Design review of the part shown in the three views and the two pictorial views. Dimensions are in mm from the part's minimum x, y and z. A direction names the side the tool comes from. Round coordinates to 2 decimals unless told otherwise and drop trailing zeros. Loops run counter-clockwise (first coordinate to the right, second up) from the corner with the lowest first, then second, coordinate; pieces in that order, holes last. Notation, with made-up numbers: M -21.5,68 L 3.5,68 A24 cw 3.5,102 Z; hole C 53,8.25 d4. An arc over 180 degrees is marked long. Return JSON: item names as keys, results as strings. Group by question number.
Q1. Clearance check with flat-ended pins moving along their axes: pin 1 Ø10 at (y, z) = (18.5, 5) entering from -X; pin 2 Ø1 at (x, z) = (5, 35.5) entering from +Y; pin 3 Ø1 at (x, z) = (3.5, 18) entering from -Y; pin 4 Ø3.5 at (y, z) = (19.65, 4.5) entering from -X. State where each tip first meets the part, or that it passes through.
Q2. Consider section D-D (z = 14). State the section outline as (x, y) points, and give its area (3 significant figures).
Q3. For the marked faces 1, 2 and 3, list the 3-axis set-ups (+Z, -Z, +X, -X, +Y, -Y) from which the entire face can be reached by the end or side of a thin tool; tool diameter is ignored.
Q4. Consider section B-B (y = 11.5). State the section outline as (x, z) points.
Q5. Consider section A-A (x = 3). State the section outline as (y, z) points (1 decimal).
Q6. Consider section C-C (y = 18.75). State the section outline as (x, z) points (1 decimal).
Q7. To check wall thickness, follow line 1 along Z through (x, y) = (4.75, 15); line 2 along Y through (x, z) = (5.5, 39) (1 decimal); line 3 along Z through (x, y) = (3.25, 22.25) (1 decimal). State the ranges of each line that lie inside material, in increasing order.
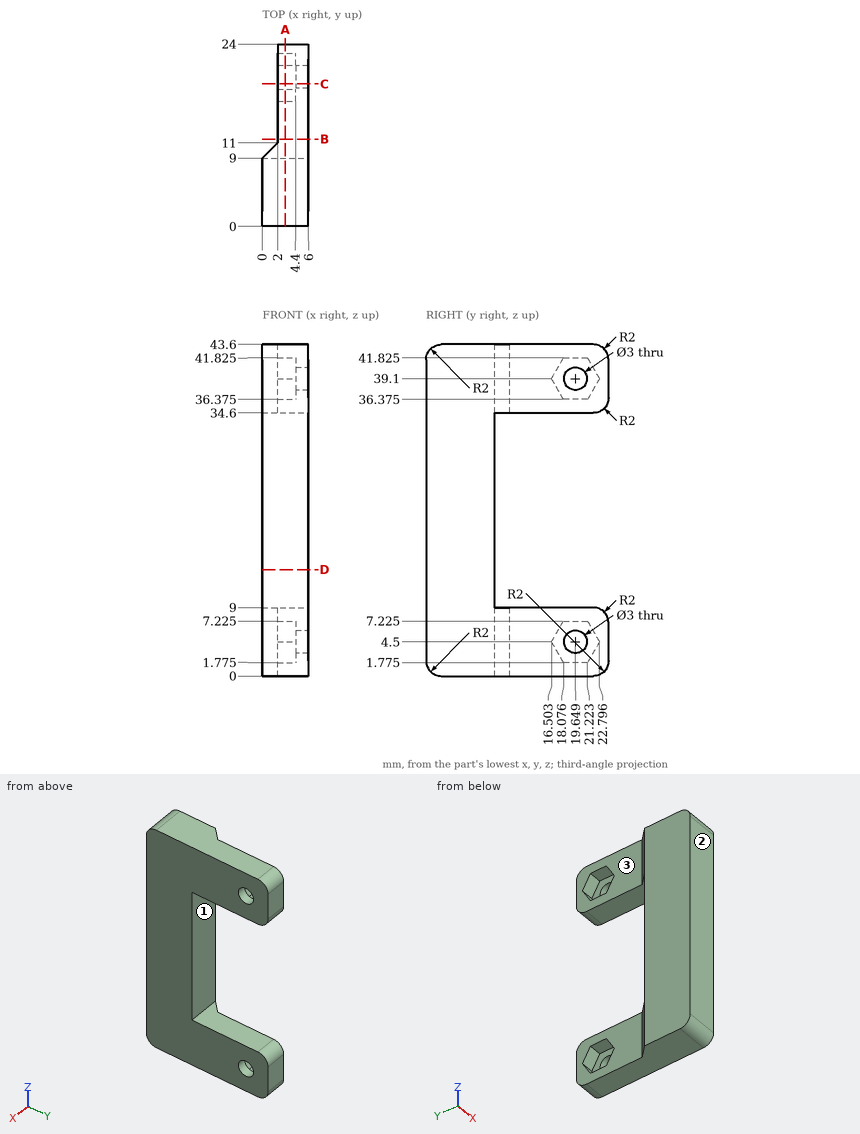
Values:
{
 "1": {"pin 1": "stops at x = 2", "pin 2": "stops at y = 23.91", "pin 3": "stops at y = 0", "pin 4": "stops at x = 4.4"},
 "2": {"outline": "M 0,0 L 6,0 L 6,9 L 0,9 Z", "area": "54.0 mm2"},
 "3": {"face 1": "+X, -X, +Y", "face 2": "+Z, -Z, +X, -X, -Y", "face 3": "+Z, -Z, -X, +Y"},
 "4": {"outline": "M 2,0 L 6,0 L 6,9 L 2,9 Z; M 2,34.6 L 6,34.6 L 6,43.6 L 2,43.6 Z"},
 "5": {"outline": "M 0,2 A2 ccw 2,0 L 22,0 A2 ccw 24,2 L 24,7 A2 ccw 22,9 L 9,9 L 9,34.6 L 22,34.6 A2 ccw 24,36.6 L 24,41.6 A2 ccw 22,43.6 L 2,43.6 A2 ccw 0,41.6 Z; hole M 16.5,4.5 L 18.1,1.8 L 21.2,1.8 L 22.8,4.5 L 21.2,7.2 L 18.1,7.2 Z; hole M 16.5,39.1 L 18.1,36.4 L 21.2,36.4 L 22.8,39.1 L 21.2,41.8 L 18.1,41.8 Z"},
 "6": {"outline": "M 2,0 L 6,0 L 6,3.3 L 4.4,3.3 L 4.4,1.8 L 2,1.8 Z; M 2,7.2 L 4.4,7.2 L 4.4,5.7 L 6,5.7 L 6,9 L 2,9 Z; M 2,34.6 L 6,34.6 L 6,37.9 L 4.4,37.9 L 4.4,36.4 L 2,36.4 Z; M 2,41.8 L 4.4,41.8 L 4.4,40.3 L 6,40.3 L 6,43.6 L 2,43.6 Z"},
 "7": {"line 1": "z = 0 to 9, 34.6 to 43.6", "line 2": "y = 0 to 18.2, 21.1 to 24", "line 3": "z = 0 to 3.6, 5.4 to 9, 34.6 to 38.2, 40 to 43.6"}
}
